For this review, take the finished solid that the model builds, in its own axes (mm). Face numbers are marked on the shaded views. A direction names the side the tool comes from. Coordinates: 2 decimals unless noted, no trailing zeros. Loops run counter-clockwise (first coordinate to the right, second up) from the corner with the lowest first, then second, coordinate; pieces in that order, holes last. Notation, with made-up numbers: (15.5, 35) -> (41.5, 35) arc R23 ccw to (41.5, 48) -> close; hole circle Ø5 at (3, 62). An arc over 180 degrees is marked (long way). Use a Markdown table: item, result.
from build123d import *
from OCP.BRepAlgoAPI import BRepAlgoAPI_Cut
from OCP.TopTools import TopTools_ListOfShape

# Parameters (mm, degrees)
BOSS_EXTRUDE1_DEPTH      = 5.73
BOSS_EXTRUDE1_DEPTH_BACK = 5.73
BOSS_EXTRUDE5_DEPTH      = 11.46
BOSS_EXTRUDE8_DEPTH      = 11.46
BOSS_EXTRUDE9_DEPTH      = 3
SKETCH11_R               = 3.54
CUT_EXTRUDE1_DEPTH       = 3
BOSS_EXTRUDE10_DEPTH     = 3
SKETCH13_R               = 1.5
CUT_EXTRUDE2_DEPTH       = 3
CUT_EXTRUDE3_START       = -3.000002
SKETCH15_R               = 1.5
CUT_EXTRUDE3_DEPTH       = 3.000002


with BuildPart() as part:
    # Sketch1 → Boss-Extrude1 (new, two sides: drawn at the far end of the back side and taken through both)
    with BuildSketch(Plane.XY.offset(-BOSS_EXTRUDE1_DEPTH_BACK)):
        Polygon((23.736099909, 38.996836219), (26.736100401, 35.996833865), (26.736100401, 3.776835326), (23.736098978, 0.776835766), (20.736098486, 3.77683812), (23.736098978, 6.776836749), (23.736098978, 32.99683803), (20.736100349, 35.996838521), align=None)
    extrude(amount=BOSS_EXTRUDE1_DEPTH + BOSS_EXTRUDE1_DEPTH_BACK)

    # Sketch6 → Boss-Extrude5 (add)
    with BuildSketch(Plane.XY.offset(5.73)):
        Polygon((20.736098486, 3.77683812), (8.576098486, 3.77683812), (8.576098486, 0.776835766), (20.736098486, 0.776835766), (23.736098978, 0.776835766), align=None)
    extrude(amount=-BOSS_EXTRUDE5_DEPTH)

    # Sketch8 → Boss-Extrude8 (add)
    with BuildSketch(Plane.XY.offset(5.73)):
        Polygon((20.736100349, 38.996836219), (23.736099909, 38.996836219), (20.736100349, 35.996838521), (8.576100349, 35.996838521), (8.576100349, 38.996836219), align=None)
    extrude(amount=-BOSS_EXTRUDE8_DEPTH)

    # Sketch9 → Boss-Extrude9 (add)
    with BuildSketch(Plane(origin=(0, 38.996836219, 0), x_dir=(1, 0, 0), z_dir=(0, 1, 0))):
        with BuildLine():
            Line((8.576100349, 5.73), (8.576100349, -5.73))
            ThreePointArc((8.576100349, -5.73), (-3.635159989, 0), (8.576100349, 5.73))
        make_face()
    extrude(amount=-BOSS_EXTRUDE9_DEPTH)

    # Sketch11 → Cut-Extrude1 (cut)
    with BuildSketch(Plane(origin=(0, 38.996836219, 0), x_dir=(1, 0, 0), z_dir=(0, 1, 0))):
        with Locations(Location((3.814840011, 0, 0), (0, 0, 270))):
            Circle(SKETCH11_R)
    extrude(amount=-CUT_EXTRUDE1_DEPTH, mode=Mode.SUBTRACT)

    # Sketch12 → Boss-Extrude10 (add)
    with BuildSketch(Plane(origin=(0, 0.776835766, 0), x_dir=(-1, 0, 0), z_dir=(0, -1, 0))):
        with BuildLine():
            Line((-8.576098486, 5.73), (-3.793078174, 5.73))
            ThreePointArc((-3.793078174, 5.73), (1.936921826, 0), (-3.793078174, -5.73))
            Line((-3.793078174, -5.73), (-8.576098486, -5.73))
            Line((-8.576098486, -5.73), (-8.576098486, 5.73))
        make_face()
    extrude(amount=-BOSS_EXTRUDE10_DEPTH)


with BuildPart() as cut_extrude2_tool:
    # Sketch13 → Cut-Extrude2 (new body)
    with BuildSketch(Plane(origin=(0, 3.77683812, 0), x_dir=(1, 0, 0), z_dir=(0, 1, 0))):
        with Locations(Location((3.81, 0, 0), (0, 0, 180))):
            Circle(SKETCH13_R)
    extrude(amount=-CUT_EXTRUDE2_DEPTH)


with BuildPart() as part_1:
    add(part.part)

    # Cut-Extrude2: cut by cut_extrude2_tool, with a tolerance
    cut_extrude2_stock = TopTools_ListOfShape()
    cut_extrude2_stock.Append(part_1.part.wrapped)
    cut_extrude2_tools = TopTools_ListOfShape()
    cut_extrude2_tools.Append(cut_extrude2_tool.part.wrapped)
    cut_extrude2_cut = BRepAlgoAPI_Cut()
    cut_extrude2_cut.SetArguments(cut_extrude2_stock)
    cut_extrude2_cut.SetTools(cut_extrude2_tools)
    cut_extrude2_cut.SetFuzzyValue(0.00001)
    cut_extrude2_cut.Build()
    add(Compound.cast(cut_extrude2_cut.Shape()).solids(), mode=Mode.REPLACE)

    # Sketch15 → Cut-Extrude3 (cut)
    with BuildSketch(Plane(origin=(26.736100401, 0, 0), x_dir=(0, 0, -1), z_dir=(1, 0, 0)).offset(CUT_EXTRUDE3_START)):
        with Locations(Location((0, 27.886833865, 0), (0, 0, 90))):
            Circle(SKETCH15_R)
        with Locations(Location((0, 19.756835766, 0), (0, 0, 90))):
            Circle(SKETCH15_R)
    extrude(amount=CUT_EXTRUDE3_DEPTH, mode=Mode.SUBTRACT)


solid = part_1.part
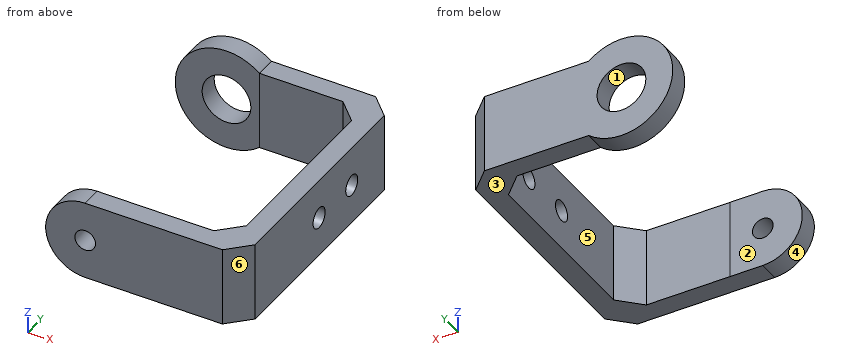
(1) Take a section at B-B on x = 17. Write out the cut boundary in (y, z).
Found:
| item | result |
|---|---|
| outline | (0.78, -5.73) -> (3.78, -5.73) -> (3.78, 5.73) -> (0.78, 5.73) -> close; (36, -5.73) -> (39, -5.73) -> (39, 5.73) -> (36, 5.73) -> close |
(2) For the marked faces 4, 5 and 6, list the 3-axis set-ups (+Z, -Z, +X, -X, +Y, -Y) from which the entire face can be reached by the end or side of a thin tool; tool diameter is ignored.
Found:
| item | result |
|---|---|
| face 4 | -X, -Y |
| face 5 | +Z, -Z, -X |
| face 6 | +Z, -Z, +X, -Y |
(3) Take a section at C-C on y = 27.5. Write out the cut boundary in (x, z), plus the area to 3 significant figures.
Found:
| item | result |
|---|---|
| outline | (23.74, -5.73) -> (26.74, -5.73) -> (26.74, -1.45) -> (23.74, -1.45) -> close; (23.74, 1.45) -> (26.74, 1.45) -> (26.74, 5.73) -> (23.74, 5.73) -> close |
| area | 25.7 mm^2 |
(4) For line 1 along Y through (x, z) = (20, -3.5); line 2 along X through (y, z) = (30, -1); line 3 along Z through (x, y) = (3, 3), list the stretches that pass through material, from the lowest coordinate up.
Found:
| item | result |
|---|---|
| line 1 | y = 0.78 to 3.78, 36 to 39 |
| line 2 | x = 23.74 to 26.74 |
| line 3 | z = -5.67 to -1.26, 1.26 to 5.67 |
(5) Mouldability with a two-part tool opening along Z and no side actions: class the marked faces 1, 2 and 3 as pulls with the +Z half, pulls with the -Z half, needs draft (parallel to the pull), parting line crosses it, or undercut.
Found:
| item | result |
|---|---|
| face 1 | undercut |
| face 2 | needs draft |
| face 3 | pulls with the -Z half |
(6) For pin 1 Ø5 at (y, z) = (27.89, 0) entering from -X; pin 2 Ø12 at (x, y) = (7, 8.5) entering from -Z; pin 3 Ø3 at (x, z) = (4.5, -1.5) entering from +Y; pin 4 Ø8 at (x, z) = (3.5, -3.5) entering from +Y, all flat-tipped, find the tip position at first contact; note any pin that passes through.
Found:
| item | result |
|---|---|
| pin 1 | stops at x = 23.74 |
| pin 2 | stops at z = -5.73 |
| pin 3 | stops at y = 3.78 |
| pin 4 | stops at y = 39 |
(7) Take a section at A-A on z = 0. State how many separate pieces and enclosed holes the cut face has, plus the area to 3 significant figures.
Found:
| item | result |
|---|---|
| separate pieces | 5 |
| enclosed holes | 0 |
| area | 226 mm^2 |
